Autodesk Inventor part; units mm, degrees
ref_plane "YZ Plane" through (0, 0, 0) normal (1, 0, 0) x (0, 1, 0)
ref_plane "XZ Plane" through (0, 0, 0) normal (0, 1, 0) x (-1, 0, 0)
ref_plane "XY Plane" through (0, 0, 0) normal (0, 0, 1) x (1, 0, 0)
sketch "Sketch1" plane through (0, 0, 0) normal (0, 1, 0) x (-1, 0, 0)
  line L0 (16.5, -20.5) -> (-16.5, -20.5)
  line L1 (-20.5, -16.5) -> (-20.5, 16.5)
  line L2 (-16.5, 20.5) -> (16.5, 20.5)
  line L3 (20.5, 16.5) -> (20.5, -16.5)
  line L4 (20.5, -16.5) -> (16.5, -20.5)
  line L5 (-16.5, -20.5) -> (-20.5, -16.5)
  line L6 (-20.5, 16.5) -> (-16.5, 20.5)
  line L7 (16.5, 20.5) -> (20.5, 16.5)
  point P0 (0, 0)
  point P1 (20.5, -20.5)
  point P2 (-20.5, 20.5)
  point P3 (-20.5, -20.5)
  point P4 (20.5, 20.5)
  dimension "d0" = 41
  dimension "d2" = 41
  dimension "d3" = 20.5
  dimension "d4" = 20.5
  dimension "d5" = 4
  dimension "d6" = 4
  dimension "d7" = 4
  dimension "d8" = 4
  dimension "d9" = 4
  dimension "d10" = 4
  dimension "d11" = 4
  dimension "d12" = 4
extrude "Extrusion1" add sketch "Sketch1" against normal blind 32
sketch "Sketch4" plane through (0, 0, 0) normal (0, 1, 0) x (-1, 0, 0)
  circle A0 centre (0, 0) radius 11.5
  circle A1 centre (0, 0) radius 4.75
  dimension "d24" = 23
  dimension "d26" = 9.5
extrude "Extrusion4" add sketch "Sketch4" along normal blind 2
sketch "Sketch5" plane through (0, 0, 0) normal (0, 1, 0) x (-1, 0, 0)
  circle A0 centre (0, 0) radius 2.5
  dimension "d29" = 5
extrude "Extrusion5" add sketch "Sketch5" along normal blind 20
sketch "Sketch6" plane through (0, 0, 0) normal (0, 1, 0) x (1, 0, 0)
  line L0 (-20.5, -16.5) -> (-20.5, 16.5)
  line L1 (-16.5, 20.5) -> (16.5, 20.5)
  circle A0 centre (0, 0) radius 11.5
  point P0 (-15.5, 15.5)
  point P1 (-15.5, -15.5)
  point P2 (15.5, 15.5)
  point P3 (15.5, -15.5)
  dimension "d33" = 15.5
  dimension "d34" = 15.5
  dimension "d37" = 31
  dimension "d40" = 31
hole "Hole1" at (-15.5, 0, -15.5) at (-15.5, 0, 15.5) at (15.5, 0, -15.5) at (15.5, 0, 15.5) direction (0, -1, 0) diameter 2.5 depth 8 tip angle 118
thread "Thread1"
thread "Thread2"
thread "Thread3"
thread "Thread4"
properties part number "stepper_short"
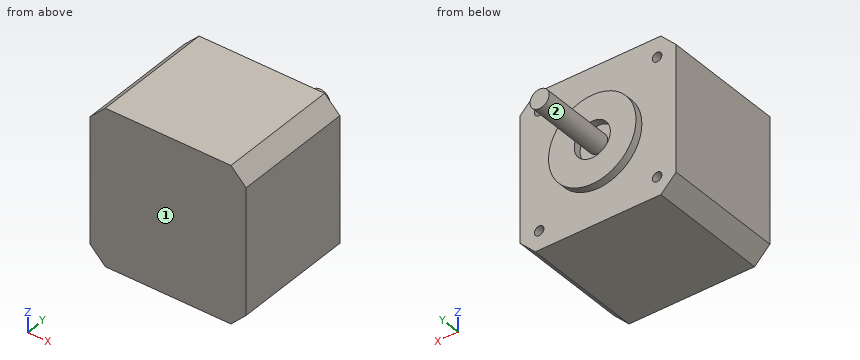
Model file for the job. Use its own axes, mm. Face numbers are marked on the shaded views. A direction names the side the tool comes from. Round coordinates to 2 decimals unless told otherwise and drop trailing zeros. Order: outer loops, then holes, each group sorted by start corner. A loop starts at its lowest first (then second) coordinate and runs counter-clockwise, first axis right, second up.
(1) Band-saw the part on A-A (x = 0). List the corners of the cut face in (y, z).
(2) 3-axis set-ups, long thin cutter, end or side, ignore diameter. For the marked faces 1 and 2: which of +Z, -Z, +X, -X, +Y, -Y reach the whole face in a straight line?
(3) Band-saw the part on B-B (y = -3.5). List the corners of the cut face in (x, z), then the cut area to 3 significant figures.
(4) Drill centre lines: line 1 (X direction, y = -4.75, z = 15.5); line 2 (Z direction, x = 15, y = -5). Where is each one in solid material? Low to high.
(5) Pin check, flat tips, straight feed: pin 1 (12 mm diameter, centred on y = 14.5, z = 7.5, fed in from -X); pin 2 (10 mm diameter, centred on y = 5.5, z = 4, fed in from +X); pin 3 (12 mm diameter, centred on x = -8, z = 14, fed in from +Y). Stop position of each tip, or through.
(6) Band-saw the part on D-D (y = -24). List the corners of the cut face in (x, z).
(7) Band-saw the part on C-C (z = -1). List the corners of the cut face in (x, y).
Verdict:
1. outline: (-32, -20.5) - (0, -20.5) - (0, -11.5) - (2, -11.5) - (2, -4.75) - (0, -4.75) - (0, -2.5) - (20, -2.5) - (20, 2.5) - (0, 2.5) - (0, 4.75) - (2, 4.75) - (2, 11.5) - (0, 11.5) - (0, 20.5) - (-32, 20.5) - close
2. face 1: +Z, -Z, +X, -X, -Y
2. face 2: +Y
3. outline: (-20.5, -16.5) - (-16.5, -20.5) - (16.5, -20.5) - (20.5, -16.5) - (20.5, 16.5) - (16.5, 20.5) - (-16.5, 20.5) - (-20.5, 16.5) - close; hole circle Ø2.5 at (-15.5, -15.5); hole circle Ø2.5 at (-15.5, 15.5); hole circle Ø2.5 at (15.5, -15.5); hole circle Ø2.5 at (15.5, 15.5)
3. area: 1,630 mm2
4. line 1: x = -20.5 to -16.75, -14.25 to 14.25, 16.75 to 20.5
4. line 2: z = -20.5 to -16.65, -14.35 to 14.35, 16.65 to 20.5
5. pin 1: stops at x = -2
5. pin 2: stops at x = 11.49
5. pin 3: stops at y = 2
6. outline: (-20.5, -16.5) - (-16.5, -20.5) - (16.5, -20.5) - (20.5, -16.5) - (20.5, 16.5) - (16.5, 20.5) - (-16.5, 20.5) - (-20.5, 16.5) - close
7. outline: (-20.5, -32) - (20.5, -32) - (20.5, 0) - (11.46, 0) - (11.46, 2) - (4.64, 2) - (4.64, 0) - (2.29, 0) - (2.29, 20) - (-2.29, 20) - (-2.29, 0) - (-4.64, 0) - (-4.64, 2) - (-11.46, 2) - (-11.46, 0) - (-20.5, 0) - close
